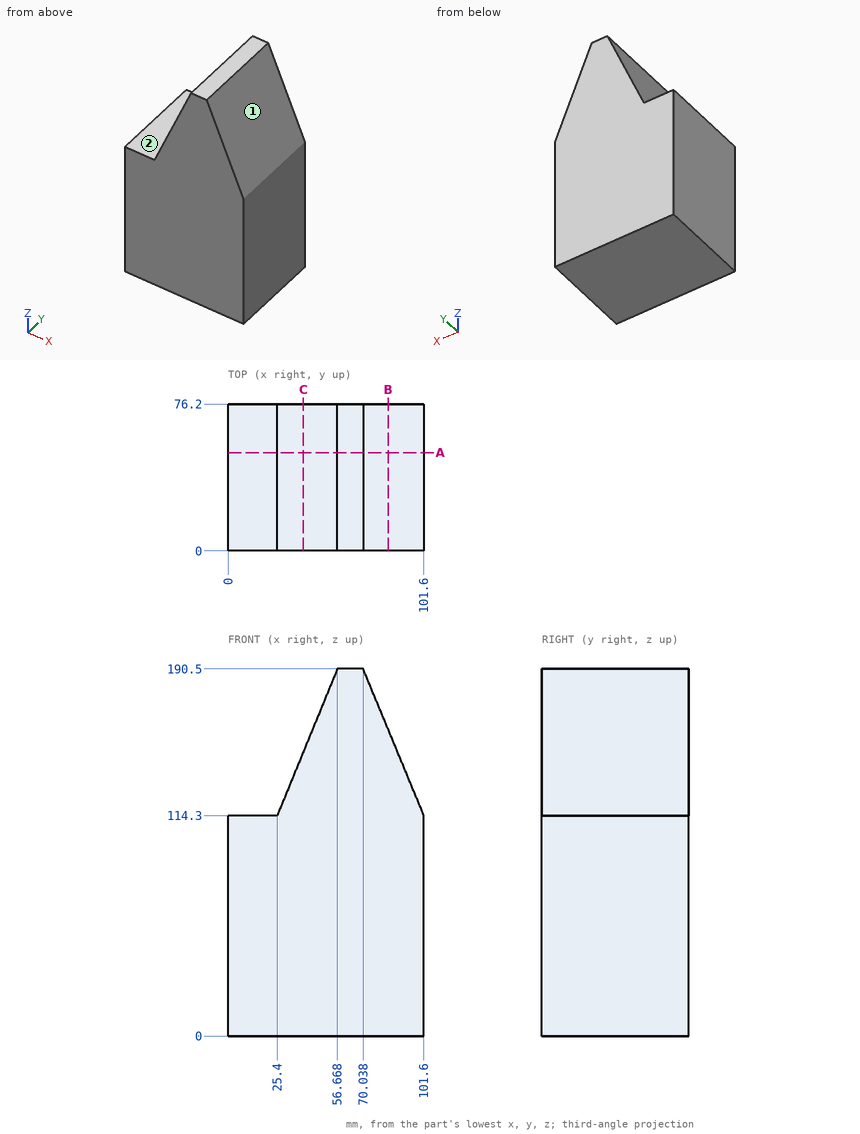
Check sheet for the drawn part. Datum: minimum x, y, z corner. Units: mm. A direction names the side the tool comes from. Round coordinates to 2 decimals unless told otherwise and drop trailing zeros. Loops run counter-clockwise (first coordinate to the right, second up) from the corner with the lowest first, then second, coordinate; pieces in that order, holes last. Notation, with made-up numbers: (7.25, 84) - (18.25, 84) arc R19 cw to (18.25, 116) - close; hole circle Ø6 at (-13, -16.5). An arc over 180 degrees is marked (long way). Write item = value, one per line. Start each with the question number.
1. Set-up check for the marked faces 1 and 2: record each of +Z, -Z, +X, -X, +Y, -Y from which the full face is reachable in a straight line by a thin tool's end or side.
2. Section check C-C on x = 39. Enter the section's corners in (y, z).
3. Section check B-B on x = 83. Enter the section's corners in (y, z), then the cut area to 3 significant figures.
4. Section check A-A on y = 51. Enter the section's corners in (x, z).
5. Thickness scan on line 1 (Z direction, x = 19, y = 36.5); line 2 (X direction, y = 61.5, z = 153); line 3 (X direction, y = 4, z = 115.5). Record the ranges inside material, lowest first.
6. Depth check by flat-ended pin: pin 1 (4 mm diameter, centred on x = 40, y = 67, fed in from +Z) (1 decimal); pin 2 (1 mm diameter, centred on y = 66, z = 115.5, fed in from +X). Enter the tip coordinate at first touch or a pass-through.
Working result:
q1.face_1 = +Z, +X, +Y, -Y
q1.face_2 = +Z, -X, +Y, -Y
q2.outline = (0, 0) - (76.2, 0) - (76.2, 147.44) - (0, 147.44) - close
q3.outline = (0, 0) - (76.2, 0) - (76.2, 159.21) - (0, 159.21) - close
q3.area = 12,100 mm^2
q4.outline = (0, 0) - (101.6, 0) - (101.6, 114.3) - (70.04, 190.5) - (56.67, 190.5) - (25.4, 114.3) - (0, 114.3) - close
q5.line_1 = 0 to 114.3
q5.line_2 = 41.28 to 85.57
q5.line_3 = 25.89 to 101.1
q6.pin_1 = 154.8
q6.pin_2 = 101.31
